```python
from build123d import *

# Parameters (mm, degrees)
F0_R     = 17.35
F1_DEPTH = 1.5
F0_R_2   = 18.85
F2_DEPTH = 20
F3_W     = 12.5
F3_H     = 5
F4_DEPTH = 25
F6_W     = 15.35
F6_H     = 8
F6_W_2   = 12.5
F6_H_2   = 5
F8_SIZE  = 1


with BuildPart() as f1:
    # F0 (on Top) → F1 (new body)
    with BuildSketch(Plane.XY):
        Circle(F0_R)
    extrude(amount=F1_DEPTH)

    # F0 (on Top) → F2 (join)
    with BuildSketch(Plane.XY):
        Circle(F0_R_2)
        Circle(F0_R, mode=Mode.SUBTRACT)
    extrude(amount=F2_DEPTH)

    # F3 (on Front) → F4 (cut)
    with BuildSketch(Plane.XZ):
        with Locations((-11.25, 4)):
            Rectangle(F3_W, F3_H)
    extrude(amount=-F4_DEPTH, mode=Mode.SUBTRACT)

    # F6 (on offset) → F7 (join, up to the next surface of F1)
    with BuildSketch(Plane.XZ.offset(-25)):
        with Locations((-11.175, 4)):
            Rectangle(F6_W, F6_H)
        with Locations((-11.25, 4)):
            Rectangle(F6_W_2, F6_H_2, mode=Mode.SUBTRACT)
    extrude(until=Until.NEXT)

    # F8
    f8_edges = [f1.edges().sort_by_distance(p)[0] for p in [
        (12.02804, 14.513743, 0),
        (-3.5, 21.761108, 0),
        (-11.175, 25, 0),
        (-18.85, 12.5, 0),
        (0, -18.85, 0),
    ]]
    chamfer(f8_edges, length=F8_SIZE)


solid = f1.part
```
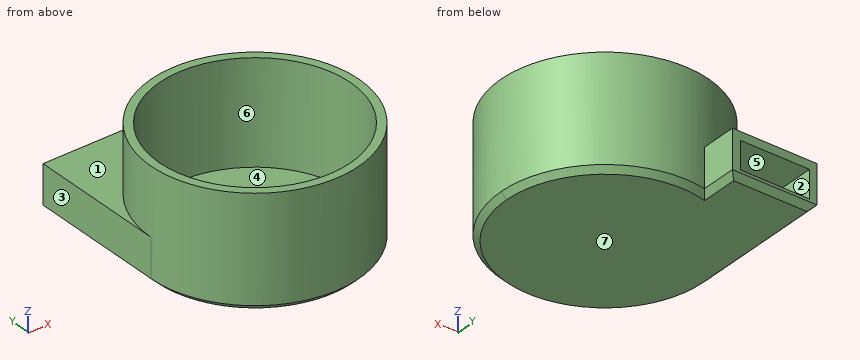
Read the model definition and answer for the solid it produces. Units are mm, in the model's axes. Face numbers are marked on the shaded views. A direction names the side the tool comes from. Round coordinates to 2 decimals unless told otherwise and drop trailing zeros. Write each loop counter-clockwise with the first axis right and the second up, starting at its lowest first coordinate (ties: lowest second). Pieces come first, ordered by that corner, then holes. Notation, with made-up numbers: (69, -20.75) - (78, -20.75) arc R31 cw to (78, 8.25) - close; hole circle Ø8 at (-1.5, 71.5). An arc over 180 degrees is marked (long way). Use CSV: the item, a comma, the result in double quotes.
Q1. Each of these flat-tipped pins is pushed along its axis until it touches: pin 1 Ø6 at (x, z) = (4, 10) entering from +Y; pin 2 Ø2 at (x, z) = (-3, 16.5) entering from +Y; pin 3 Ø1.5 at (x, z) = (-10.5, 5.5) entering from -Y. Where does it stop, or does it pass through?
Values:
pin 1,"stops at y = 18.82"
pin 2,"stops at y = 18.74"
pin 3,"stops at y = -16.13"
Q2. Straight lines are drawn through the part: line 1 along Z through (x, y) = (-10, 21); line 2 along X through (y, z) = (0, 9). For each, find the intervals that lie inside material, in ascending order.
Values:
line 1,"z = 0 to 1.5, 6.5 to 8"
line 2,"x = -18.85 to -17.35, 17.35 to 18.85"
Q3. Find section C-C, the plane z = 18.5. Write down the section's boundary in (x, y).
Values:
outline,"circle Ø37.7 at (0, 0); hole circle Ø34.7 at (0, 0)"
Q4. A tool of negligible diameter and unlimited length cuts with its end or side. For the marked faces 4, 5, 6 and 7, from which of +Z, -Z, +X, -X, +Y, -Y can it reach the whole face along a straight path? Write none if from no direction.
Values:
face 4,"none"
face 5,"+Y"
face 6,"+Z"
face 7,"-Z, +X, -X, +Y, -Y"
Q5. Find section A-A, the plane z = 4.75. Write down the section's boundary in (x, y).
Values:
outline,"(-18.85, 0) arc R18.85 ccw (long way) to (-3.5, 18.52) - (-3.5, 25) - (-5, 25) - (-5, 16.61) arc R17.35 cw (long way) to (-17.35, 0) - (-17.5, 0) - (-17.5, 25) - (-18.85, 25) - close"
Q6. Find section B-B, the plane x = 0. Write down the section's boundary in (y, z).
Values:
outline,"(-18.85, 1) - (-17.85, 0) - (17.85, 0) - (18.85, 1) - (18.85, 20) - (17.35, 20) - (17.35, 1.5) - (-17.35, 1.5) - (-17.35, 20) - (-18.85, 20) - close"
Q7. Determine the mould class of the marked faces 1, 2 and 3 for opening direction Z: +Z half, -Z half, draft (parallel to the pull), parting line (faces both ways), or undercut.
Values:
face 1,"+Z half"
face 2,"undercut"
face 3,"draft"
